```python
from build123d import *

# Parameters (mm, degrees)
AUFSATZ_LINEAR_AUSTRAGEN1_DEPTH = 25
SKIZZE2_W                       = 6
SKIZZE2_H                       = 1.8
AUFSATZ_LINEAR_AUSTRAGEN2_DEPTH = 8
VERRUNDUNG1_R                   = 0.2


with BuildPart() as part:
    # Skizze1 → Aufsatz-Linear austragen1 (new body)
    with BuildSketch(Plane.XY):
        Polygon((-4.75, 0.9), (-6.7, 0.9), (-6.7, -0.9), (-4.75, -0.9), (-4.75, -2.9), (-3.75, -2.9), (-3.75, -0.9), (3.75, -0.9), (3.75, -2.9), (4.75, -2.9), (4.75, -0.9), (6.7, -0.9), (6.7, 0.9), (4.75, 0.9), (4.75, 2.9), (3.75, 2.9), (3.75, 0.9), (-3.75, 0.9), (-3.75, 2.9), (-4.75, 2.9), align=None)
    extrude(amount=AUFSATZ_LINEAR_AUSTRAGEN1_DEPTH)

    # Skizze2 → Aufsatz-Linear austragen2 (add)
    with BuildSketch(Plane(origin=(0, 0, 0), x_dir=(-1, 0, 0), z_dir=(0, 0, -1))):
        Rectangle(SKIZZE2_W, SKIZZE2_H)
    extrude(amount=AUFSATZ_LINEAR_AUSTRAGEN2_DEPTH)

    # Verrundung1
    verrundung1_edges = [part.edges().sort_by_distance(p)[0] for p in [
        (-4.75, -1.9, 25),
        (-4.25, -2.9, 25),
        (-5.725, 0.9, 0),
        (-4.75, 1.9, 0),
        (-4.25, 2.9, 0),
        (-3.75, -1.9, 25),
        (4.25, 2.9, 0),
        (4.75, 1.9, 0),
        (5.725, 0.9, 0),
        (6.7, 0, 0),
        (5.725, -0.9, 0),
        (4.75, -1.9, 0),
        (4.25, -2.9, 0),
        (0, -0.9, 25),
        (-4.25, -2.9, 0),
        (-4.75, -1.9, 0),
        (-5.725, -0.9, 0),
        (-6.7, 0, 0),
        (3.75, -1.9, 25),
        (4.25, -2.9, 25),
        (-6.7, 0.9, 12.5),
        (-4.75, 2.9, 12.5),
        (-3.75, 2.9, 12.5),
        (3.75, 2.9, 12.5),
        (4.75, 2.9, 12.5),
        (6.7, 0.9, 12.5),
        (6.7, -0.9, 12.5),
        (4.75, -2.9, 12.5),
        (3.75, -2.9, 12.5),
        (-3.75, -2.9, 12.5),
        (-4.75, -2.9, 12.5),
        (-6.7, -0.9, 12.5),
        (4.75, -1.9, 25),
        (5.725, -0.9, 25),
        (6.7, 0, 25),
        (5.725, 0.9, 25),
        (-6.7, 0, 25),
        (4.75, 1.9, 25),
        (4.25, 2.9, 25),
        (3, 0, -8),
        (3.75, 1.9, 25),
        (0, -0.9, -8),
        (-3, 0, -8),
        (0, 0.9, -8),
        (0, 0.9, 25),
        (-3.75, 1.9, 25),
        (-4.25, 2.9, 25),
        (-4.75, 1.9, 25),
        (-5.725, 0.9, 25),
        (-5.725, -0.9, 25),
    ]]
    fillet(verrundung1_edges, radius=VERRUNDUNG1_R)


solid = part.part
```
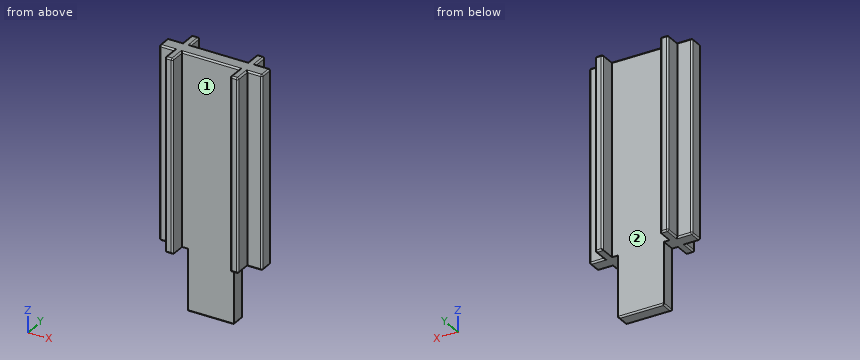
Build history of the part. All positions in model axes, mm. Face numbers are marked on the shaded views. A direction names the side the tool comes from. Give positions to 0.01 mm unless a question says otherwise; leave off trailing zeros. Loops run counter-clockwise (first coordinate to the right, second up) from the corner with the lowest first, then second, coordinate; pieces in that order, holes last.
Item 1: Flat gauge pins, fed straight in: pin 1 (4 mm diameter, centred on x = 0.5, z = 3, fed in from -Y); pin 2 (2 mm diameter, centred on x = 2, z = 10, fed in from +Y); pin 3 (6 mm diameter, centred on x = 5, z = 15, fed in from +Y); pin 4 (0.5 mm diameter, centred on y = -1.5, z = 16, fed in from +X). Where does each tip first touch, or does it go through?
Answers follow:
pin 1: stops at y = -0.9
pin 2: stops at y = 0.9
pin 3: stops at y = 2.9
pin 4: stops at x = 4.75
Item 2: Drill centre lines: line 1 (X direction, y = -2.45, z = 1.5); line 2 (Y direction, x = -2, z = -0.5); line 3 (X direction, y = 0.75, z = -2). Where is each one in solid material? Low to high.
Answers follow:
line 1: x = -4.75 to -3.75, 3.75 to 4.75
line 2: y = -0.9 to 0.9
line 3: x = -3 to 3
Item 3: Slice it at A-A, the plane y = -1.45. List the corners of the cut face in (x, z).
Answers follow:
outline: (-4.75, 0.2) arc R0.2 ccw to (-4.55, 0) - (-3.75, 0) - (-3.75, 24.8) arc R0.2 ccw to (-3.95, 25) - (-4.55, 25) arc R0.2 ccw to (-4.75, 24.8) - close; (3.75, 0) - (4.55, 0) arc R0.2 ccw to (4.75, 0.2) - (4.75, 24.8) arc R0.2 ccw to (4.55, 25) - (3.95, 25) arc R0.2 ccw to (3.75, 24.8) - close
Item 4: Slice it at B-B, the plane x = -5.25. List the corners of the cut face in (y, z).
Answers follow:
outline: (-0.9, 0.2) arc R0.2 ccw to (-0.7, 0) - (0.7, 0) arc R0.2 ccw to (0.9, 0.2) - (0.9, 24.8) arc R0.2 ccw to (0.7, 25) - (-0.7, 25) arc R0.2 ccw to (-0.9, 24.8) - close
Item 5: Which spindle directions (+Z, -Z, +X, -X, +Y, -Y) get a long thin tool onto all of the face, cutting with end or side? Do the marked faces 1 and 2. Say none if no direction does.
Answers follow:
face 1: +Z, -Z, -Y
face 2: +Z, -Z, +Y
Item 6: Slice it at D-D, the plane x = 2.5. List the corners of the cut face in (y, z), and give its area (3 significant figures).
Answers follow:
outline: (-0.9, -7.8) arc R0.2 ccw to (-0.7, -8) - (0.7, -8) arc R0.2 ccw to (0.9, -7.8) - (0.9, 24.8) arc R0.2 ccw to (0.7, 25) - (-0.7, 25) arc R0.2 ccw to (-0.9, 24.8) - close
area: 59.4 mm2
